from build123d import *

# Parameters (mm, degrees)
F1_DEPTH = 60


with BuildPart() as f1:
    # F0 (on Right) → F1 (new body)
    with BuildSketch(Plane.YZ):
        Polygon((-5, 0), (0, 0), (0, 30), (-5, 27.5), align=None)
        Polygon((-5, 27.5), (0, 30), (0, 35.59017), (-60, 5.59017), (-60, 0), (-55, 2.5), align=None)
        Polygon((-55, 0), (-55, 2.5), (-60, 0), align=None)
    extrude(amount=F1_DEPTH)


solid = f1.part
Design review of the part built by this model. Coordinates are the model's own, in mm. A direction names the side the tool comes from. Round coordinates to 2 decimals unless told otherwise and drop trailing zeros. Write each loop counter-clockwise with the first axis right and the second up, starting at its lowest first coordinate (ties: lowest second). Pieces come first, ordered by that corner, then holes.
Item 1: For faces 1 (the flat face through (30, -5, 14)), 2 (the flat face through (30, -60, 3)), list the 3-axis set-ups (+Z, -Z, +X, -X, +Y, -Y) from which the entire face can be reached by the end or side of a thin tool; tool diameter is ignored.
Item 2: For pin 1 Ø14 at (x, z) = (23, 18) entering from -Y; pin 2 Ø5 at (x, y) = (42, -11) entering from +Z; pin 3 Ø8 at (x, y) = (52.5, -27) entering from +Z, all flat-tipped, find the tip position at first contact; note any pin that passes through.
Item 3: Consider section B-B on x = 29.5. Give the boundary of the cut face in (y, z).
Item 4: Draft analysis for pull direction Y (two halves, no side actions). For faces 3 (the flat face through (30, -55, 1)), 4 (the flat face through (30, 0, 18)), 5 (the flat face through (60, -23, 19)), 6 (the flat face through (29.58, -29.58, 20.8)), state which applies: released by +Y, released by -Y, zero draft, split by the parting line, or undercut.
Item 5: Consider section D-D on z = 32.5. Give the boundary of the cut face in (x, y).
Item 6: Consider section C-C on y = -12. Give the boundary of the cut face in (x, z), and give its area (3 significant figures).
Item 7: Wall thickness on L1, parallel to Y at x = 7, z = 2.5; L2, parallel to Y at x = 36, z = 23; L3, parallel to Z at x = 3, y = -19.5: over which ranges is each line inside the solid? List them lowest first.
Item 8: Consider section A-A on z = 21. Give the boundary of the cut face in (x, y), and give its area (3 significant figures).
Check values:
1. face 1: -Z, +X, -X
1. face 2: +Z, -Z, +X, -X, -Y
2. pin 1: stops at y = -49.18
2. pin 2: stops at z = 31.34
2. pin 3: stops at z = 24.09
3. outline: (-60, 0) - (-55, 0) - (-55, 2.5) - (-5, 27.5) - (-5, 0) - (0, 0) - (0, 35.59) - (-60, 5.59) - close
4. face 3: undercut
4. face 4: released by +Y
4. face 5: zero draft
4. face 6: released by -Y
5. outline: (0, -6.18) - (60, -6.18) - (60, 0) - (0, 0) - close
6. outline: (0, 24) - (60, 24) - (60, 29.59) - (0, 29.59) - close
6. area: 335 mm2
7. L1: y = -60 to -55, -5 to 0
7. L2: y = -25.18 to -14, -5 to 0
7. L3: z = 20.25 to 25.84
8. outline: (0, -29.18) - (60, -29.18) - (60, -18) - (0, -18) - close; (0, -5) - (60, -5) - (60, 0) - (0, 0) - close
8. area: 971 mm2
